The listing builds one solid part. Answer for the finished solid, in the listing's coordinates (mm). Coordinates: 2 decimals unless noted, no trailing zeros. Write each loop counter-clockwise with the first axis right and the second up, starting at its lowest first coordinate (ties: lowest second). Pieces come first, ordered by that corner, then holes. Notation, with made-up numbers: M 44,85.5 L 76,85.5 A21 cw 76,89.5 Z; hole C 49.25,-30.5 d2. An arc over 180 degrees is marked long. Answer as CSV lines item,"result". Start each with the question number.
```python
from build123d import *

# Parameters (mm, degrees)
SKETCH2_W           = 145
SKETCH2_H           = 82.2
SKETCH2_R           = 1.25
SKETCH2_R_2         = 1.5
SKETCH2_R_3         = 3.25
SKETCH2_R_4         = 3.5
SKETCH2_W_2         = 19.4
SKETCH2_H_2         = 12.9
SKETCH2_W_3         = 59.1
SKETCH2_H_3         = 31.49
BOSS_EXTRUDE1_DEPTH = 1


with BuildPart() as part:
    # Sketch2 → Boss-Extrude1 (new body)
    with BuildSketch(Plane(origin=(0, 0, 0), x_dir=(1, 0, 0), z_dir=(0, 1, 0))):
        Rectangle(SKETCH2_W, SKETCH2_H)
        with Locations(Location((-68.25, -36.85, 0), (0, 0, 270))):
            Circle(SKETCH2_R, mode=Mode.SUBTRACT)
        with Locations(Location((68.25, -36.85, 0), (0, 0, 270))):
            Circle(SKETCH2_R, mode=Mode.SUBTRACT)
        with Locations(Location((-10, -21.4, 0), (0, 0, 270))):
            Circle(SKETCH2_R_2, mode=Mode.SUBTRACT)
        with Locations(Location((30, -21.4, 0), (0, 0, 270))):
            Circle(SKETCH2_R_2, mode=Mode.SUBTRACT)
        with Locations(Location((-15, -21.4, 0), (0, 0, 270))):
            Circle(SKETCH2_R_2, mode=Mode.SUBTRACT)
        with Locations(Location((25, -21.4, 0), (0, 0, 270))):
            Circle(SKETCH2_R_2, mode=Mode.SUBTRACT)
        with Locations(Location((-12.5, -12.9, 0), (0, 0, 270))):
            Circle(SKETCH2_R_3, mode=Mode.SUBTRACT)
        with Locations(Location((-46, 12.1, 0), (0, 0, 270))):
            Circle(SKETCH2_R_3, mode=Mode.SUBTRACT)
        with Locations(Location((46, 12.1, 0), (0, 0, 270))):
            Circle(SKETCH2_R_4, mode=Mode.SUBTRACT)
        with Locations(Location((-68.25, 36.85, 0), (0, 0, 270))):
            Circle(SKETCH2_R, mode=Mode.SUBTRACT)
        with Locations(Location((68.25, 36.85, 0), (0, 0, 270))):
            Circle(SKETCH2_R, mode=Mode.SUBTRACT)
        with Locations(Location((-66, 12.1, 0), (0, 0, 270))):
            Circle(SKETCH2_R, mode=Mode.SUBTRACT)
        with Locations(Location((-50, 34.1, 0), (0, 0, 270))):
            Circle(SKETCH2_R, mode=Mode.SUBTRACT)
        with Locations(Location((66, 12.1, 0), (0, 0, 90))):
            Circle(SKETCH2_R, mode=Mode.SUBTRACT)
        with Locations(Location((50, 34.1, 0), (0, 0, 90))):
            Circle(SKETCH2_R, mode=Mode.SUBTRACT)
        with Locations(Location((27.5, -12.9, 0), (0, 0, 270))):
            Circle(SKETCH2_R_3, mode=Mode.SUBTRACT)
        with BuildLine():
            Line((3.425, -33.859530524), (3.425, -34.9))
            Line((3.425, -34.9), (6.575, -34.9))
            Line((6.575, -34.9), (6.575, -33.859530524))
            ThreePointArc((6.575, -33.859530524), (5, -16.2), (3.425, -33.859530524))
        make_face(mode=Mode.SUBTRACT)
        with BuildLine():
            Line((43.425, -34.9), (43.425, -33.859530524))
            ThreePointArc((43.425, -33.859530524), (45, -16.2), (46.575, -33.859530524))
            Line((46.575, -33.859530524), (46.575, -34.9))
            Line((46.575, -34.9), (43.425, -34.9))
        make_face(mode=Mode.SUBTRACT)
        with Locations((-47, -24.65)):
            Rectangle(SKETCH2_W_2, SKETCH2_H_2, mode=Mode.SUBTRACT)
        with Locations((0, 9.455)):
            Rectangle(SKETCH2_W_3, SKETCH2_H_3, mode=Mode.SUBTRACT)
    extrude(amount=BOSS_EXTRUDE1_DEPTH)


solid = part.part
```
1) The part is cut by section B-B (x = 5). Determine the outline of the cut face in (y, z).
2) The part is cut by section A-A (z = 12.9). Determine the outline of the cut face in (x, y), then the cut area to 3 significant figures.
3) For a pull along X with two mould halves and no side action, classify faces 1 (the face through (-14.55, 0.49, 22.83)), 2 (the face through (-1, 0, 9)), 3 (the face through (-10.575, 0.493, 22.786)) as +X half, -X half, draft (parallel to the pull), parting line (faces both ways), or undercut.
4) The part is cut by section C-C (z = -2). Determine the outline of the cut face in (x, y).
5) This flat-tipped pin is pushed along its axis until it touches: P1, Ø4, axis at x = -46, z = -12.1, coming from the -Y side. Where does it stop, or does it pass through?
6) The part is cut by section D-D (y = 0.5). Count the separate pieces of the cut face and the enclosed holes in it, then the cut area to 3 significant figures.
7) Find the intervals of material crossed by line 1 (X direction, y = 0.4, z = -36.85); line 2 (X direction, y = 0.55, z = -34.1); line 3 (Z direction, x = 68.25, y = 0.7), in increasing order. Write a range as from..to.
Completed:
1,outline,"M 0,-41.1 L 1,-41.1 L 1,-25.2 L 0,-25.2 Z; M 0,6.29 L 1,6.29 L 1,16.2 L 0,16.2 Z; M 0,34.9 L 1,34.9 L 1,41.1 L 0,41.1 Z"
2,outline,"M -72.5,0 L -15.75,0 L -15.75,1 L -72.5,1 Z; M -9.25,0 L 24.25,0 L 24.25,1 L -9.25,1 Z; M 30.75,0 L 72.5,0 L 72.5,1 L 30.75,1 Z"
2,area,"132 mm²"
3,face 1,"undercut"
3,face 2,"draft"
3,face 3,"undercut"
4,outline,"M -72.5,0 L -29.55,0 L -29.55,1 L -72.5,1 Z; M 29.55,0 L 72.5,0 L 72.5,1 L 29.55,1 Z"
5,P1,"through"
6,separate pieces,"1"
6,enclosed holes,"20"
6,area,"9,100 mm²"
7,line 1,"-72.5..-69.5, -67..67, 69.5..72.5"
7,line 2,"-72.5..-51.25, -48.75..48.75, 51.25..72.5"
7,line 3,"-41.1..-38.1, -35.6..35.6, 38.1..41.1"
